from build123d import *

# Parameters (mm, degrees)
SKETCH_1_W                   = 600
SKETCH_1_H                   = 12
EXTRUDE_1_DEPTH              = 8
CUT_EXTRUDE_1_DEPTH          = 601.043331769
CUT_EXTRUDE_2_DEPTH          = 601.043331769
CUT_EXTRUDE_3_DEPTH          = 601.043331769
CUT_EXTRUDE_4_DEPTH          = 601.043331769
CUT_EXTRUDE_5_DEPTH          = 601.043331769
CUT_EXTRUDE_6_DEPTH          = 601.043331769
HOLE_WIZARD_M3_1_D           = 3.5
HOLE_WIZARD_M3_1_CBORE_D     = 5.9999
HOLE_WIZARD_M3_1_CBORE_DEPTH = 4.5
CHAMFER_1_SIZE               = 0.6
FILLET_1_R                   = 0.2


with BuildPart() as part:
    # 草图1 → 凸台-拉伸1 (new body)
    with BuildSketch(Plane(origin=(0, 4, 0), x_dir=(1, 0, 0), z_dir=(0, 1, 0))):
        Rectangle(SKETCH_1_W, SKETCH_1_H)
    extrude(amount=-EXTRUDE_1_DEPTH)

    # 草图2 → 切除-拉伸1 (cut, through all)
    with BuildSketch(Plane(origin=(300, 0, 0), x_dir=(0, 0, -1), z_dir=(1, 0, 0))):
        with BuildLine():
            Line((6, 1.51), (6, 2.01))
            Line((6, 2.01), (4.8, 2.01))
            ThreePointArc((4.8, 2.01), (4.55, 1.76), (4.8, 1.51))
            Line((4.8, 1.51), (6, 1.51))
        make_face()
    extrude(amount=-CUT_EXTRUDE_1_DEPTH, mode=Mode.SUBTRACT)

    # 草图3 → 切除-拉伸2 (cut, through all)
    with BuildSketch(Plane(origin=(300, 0, 0), x_dir=(0, 0, -1), z_dir=(1, 0, 0))):
        with BuildLine():
            Line((6, 2.01), (6, 3.111111))
            ThreePointArc((6, 3.111111), (5.367595703, 2.693428684), (5.04, 2.01))
            Line((5.04, 2.01), (6, 2.01))
        make_face()
    extrude(amount=-CUT_EXTRUDE_2_DEPTH, mode=Mode.SUBTRACT)

    # 草图4 → 切除-拉伸3 (cut, through all)
    with BuildSketch(Plane(origin=(300, 0, 0), x_dir=(0, 0, -1), z_dir=(1, 0, 0))):
        with BuildLine():
            Line((6, 1.51), (5.04, 1.51))
            ThreePointArc((5.04, 1.51), (5.367595703, 0.826571316), (6, 0.408889))
            Line((6, 0.408889), (6, 1.51))
        make_face()
    extrude(amount=-CUT_EXTRUDE_3_DEPTH, mode=Mode.SUBTRACT)

    # 草图5 → 切除-拉伸4 (cut, through all)
    with BuildSketch(Plane(origin=(300, 0, 0), x_dir=(0, 0, -1), z_dir=(1, 0, 0))):
        with BuildLine():
            Line((-6, 2.01), (-6, 1.51))
            Line((-6, 1.51), (-4.8, 1.51))
            ThreePointArc((-4.8, 1.51), (-4.55, 1.76), (-4.8, 2.01))
            Line((-4.8, 2.01), (-6, 2.01))
        make_face()
    extrude(amount=-CUT_EXTRUDE_4_DEPTH, mode=Mode.SUBTRACT)

    # 草图6 → 切除-拉伸5 (cut, through all)
    with BuildSketch(Plane(origin=(300, 0, 0), x_dir=(0, 0, -1), z_dir=(1, 0, 0))):
        with BuildLine():
            Line((-6, 1.51), (-6, 0.408889))
            ThreePointArc((-6, 0.408889), (-5.367595703, 0.826571316), (-5.04, 1.51))
            Line((-5.04, 1.51), (-6, 1.51))
        make_face()
    extrude(amount=-CUT_EXTRUDE_5_DEPTH, mode=Mode.SUBTRACT)

    # 草图7 → 切除-拉伸6 (cut, through all)
    with BuildSketch(Plane(origin=(300, 0, 0), x_dir=(0, 0, -1), z_dir=(1, 0, 0))):
        with BuildLine():
            Line((-6, 2.01), (-5.04, 2.01))
            ThreePointArc((-5.04, 2.01), (-5.367595703, 2.693428684), (-6, 3.111111))
            Line((-6, 3.111111), (-6, 2.01))
        make_face()
    extrude(amount=-CUT_EXTRUDE_6_DEPTH, mode=Mode.SUBTRACT)

    # M3 六角头机械螺钉的柱形沉头孔1 (through all)
    with Locations(Plane(origin=(0, 4, 0), x_dir=(1, 0, 0), z_dir=(0, 1, 0))):
        with Locations((-287.5, 0), (-262.5, 0), (-237.5, 0), (-212.5, 0), (-187.5, 0), (-162.5, 0), (-137.5, 0), (-112.5, 0), (-87.5, 0), (-62.5, 0), (-37.5, 0), (-12.5, 0), (12.5, 0), (37.5, 0), (62.5, 0), (87.5, 0), (112.5, 0), (137.5, 0), (162.5, 0), (187.5, 0), (212.5, 0), (237.5, 0), (262.5, 0), (287.5, 0)):
            CounterBoreHole(HOLE_WIZARD_M3_1_D / 2, HOLE_WIZARD_M3_1_CBORE_D / 2, HOLE_WIZARD_M3_1_CBORE_DEPTH)

    # 倒角1
    chamfer_1_edges = [part.edges().sort_by_distance(p)[0] for p in [
        (0, -4, -6),
        (0, -4, 6),
    ]]
    chamfer(chamfer_1_edges, length=CHAMFER_1_SIZE)

    # 圆角1
    fillet_1_edges = [part.edges().sort_by_distance(p)[0] for p in [
        (0, 2.01, -5.04),
        (0, 3.111111, -6),
        (0, 0.408889, -6),
        (0, 1.51, -5.04),
        (0, 4, -6),
        (0, 4, 6),
        (0, 1.51, 5.04),
        (0, 0.408889, 6),
        (0, 3.111111, 6),
        (0, 2.01, 5.04),
    ]]
    fillet(fillet_1_edges, radius=FILLET_1_R)


solid = part.part
Geometry check sheet. Reference: the model listing, model coordinates, mm. Give positions to 0.01 mm unless a question says otherwise; leave off trailing zeros. Order: outer loops, then holes, each group sorted by start corner. A loop starts at its lowest first (then second) coordinate and runs counter-clockwise, first axis right, second up. Notation, with made-up numbers: (6.25, 5) - (11.25, 5) arc R30 ccw to (11.25, 37) - close; hole circle Ø11 at (-25.75, 74.25). An arc over 180 degrees is marked (long way). Answer as a JSON object with one key per item and string values.
(1) Cross-section at A-A (x = -171). Record the cut outline in (y, z).
Report:
{"outline": "(-4, -5.4) - (-3.4, -6) - (0.27, -6) arc R0.2 ccw to (0.45, -5.88) arc R1.42 cw to (1.37, -5.07) arc R0.2 ccw to (1.51, -4.88) - (1.51, -4.8) arc R0.25 cw to (2.01, -4.8) - (2.01, -4.88) arc R0.2 ccw to (2.15, -5.07) arc R1.42 cw to (3.07, -5.88) arc R0.2 ccw to (3.25, -6) - (3.8, -6) arc R0.2 ccw to (4, -5.8) - (4, 5.8) arc R0.2 ccw to (3.8, 6) - (3.25, 6) arc R0.2 ccw to (3.07, 5.88) arc R1.42 cw to (2.15, 5.07) arc R0.2 ccw to (2.01, 4.88) - (2.01, 4.8) arc R0.25 cw to (1.51, 4.8) - (1.51, 4.88) arc R0.2 ccw to (1.37, 5.07) arc R1.42 cw to (0.45, 5.88) arc R0.2 ccw to (0.27, 6) - (-3.4, 6) - (-4, 5.4) - close"}
(2) Material ranges on line 1 (Z direction, x = -37.5, y = 0.85); line 2 (Z direction, x = 62.5, y = -1.6); line 3 (Y direction, x = -205, z = -5), recorded low to high.
Report:
{"line 1": "-5.35 to -3, 3 to 5.35", "line 2": "-6 to -1.75, 1.75 to 6", "line 3": "-4 to 1.47, 2.05 to 4"}
(3) Depth check by flat-ended pin: pin 1 Ø3 at (x, z) = (-188, 0) entering from +Y; pin 2 Ø3 at (x, z) = (12.5, 0) entering from -Y. Enter the tip coordinate at first touch or a pass-through.
Report:
{"pin 1": "y = -0.5", "pin 2": "through"}
